```python
from build123d import *

# Parameters (mm, degrees)
F0_W      = 356
F0_H      = 100
F1_DEPTH  = 5
F2_R      = 5
F2_R_2    = 12.5
F3_DEPTH  = 5.001
F4_R      = 1.5
F5_DEPTH  = 5.001
F6_W      = 49.406879
F6_H      = 21.095738
F7_DEPTH  = 25
F9_W      = 63.062
F9_H      = 100
F10_DEPTH = 5
F11_R     = 3
F12_DEPTH = 25
F13_W     = 419.062
F13_H     = 5
F14_DEPTH = 70


with BuildPart() as f1:
    # F0 (on Top) → F1 (new body)
    with BuildSketch(Plane.XY):
        Rectangle(F0_W, F0_H)
    extrude(amount=F1_DEPTH)

    # F2 (on face) → F3 (cut, through all)
    with BuildSketch(Plane.XY.offset(5)):
        with Locations((-155, 37.335402)):
            Circle(F2_R)
        with Locations((155, 37.335402)):
            Circle(F2_R)
        with Locations((-48.086096, 0)):
            Circle(F2_R_2)
        with Locations((51.913904, 0)):
            Circle(F2_R_2)
    extrude(amount=-F3_DEPTH, mode=Mode.SUBTRACT)

    # F4 (on face) → F5 (cut, through all)
    with BuildSketch(Plane.XY.offset(5)):
        with Locations((0, 2.148001)):
            Circle(F4_R)
        with Locations((100, 2.148001)):
            Circle(F4_R)
        with Locations((-100, 2.148001)):
            Circle(F4_R)
    extrude(amount=-F5_DEPTH, mode=Mode.SUBTRACT)

    # F9 (on Top) → F10 (join, through all)
    with BuildSketch(Plane.XY):
        with Locations((-209.531, 0)):
            Rectangle(F9_W, F9_H)
    extrude(amount=F10_DEPTH)

    # F11 (on face) → F12 (cut)
    with BuildSketch(Plane.XY.offset(5)):
        with Locations((-223.56236, -20)):
            Circle(F11_R)
        with Locations((-223.56236, -40)):
            Circle(F11_R)
    extrude(amount=-F12_DEPTH, mode=Mode.SUBTRACT)

    # F13 (on face) → F14 (join)
    with BuildSketch(Plane(origin=(0, 0, 0), x_dir=(1, 0, 0), z_dir=(0, 0, -1))):
        with Locations((-31.531, -52.5)):
            Rectangle(F13_W, F13_H)
    extrude(amount=-F14_DEPTH)


with BuildPart() as f7:
    # F6 (on Top) → F7 (new body)
    with BuildSketch(Plane.XY):
        with Locations((37.024449, 48.380569)):
            Rectangle(F6_W, F6_H)
    extrude(amount=F7_DEPTH)


solid = f1.part
```
The listing builds one solid part. Answer for the finished solid, in the listing's coordinates (mm). A direction names the side the tool comes from. Give positions to 0.01 mm unless a question says otherwise; leave off trailing zeros. Write each loop counter-clockwise with the first axis right and the second up, starting at its lowest first coordinate (ties: lowest second). Pieces come first, ordered by that corner, then holes. Notation, with made-up numbers: (-1, 44) -> (53, 44) arc R28 ccw to (53, 67) -> close; hole circle Ø7 at (74, 59). An arc over 180 degrees is marked (long way). Write item = value, one per line. Start each with the question number.
1) Which of the six approach directions +Z, -Z, +X, -X, +Y, -Y give full straight-line access (tool end or side, diameter ignored) to faces 4 (the face through (-34, 1, 5)), 5 (the face through (-241.062, 18, 4))?
2) The part is cut by section C-C, the plane y = -33. Determine the outline of the cut face in (x, z), and give its area (3 significant figures).
3) The part is cut by section A-A, the plane x = -155. Determine the outline of the cut face in (y, z), and give its area (3 significant figures).
4) The part is cut by section B-B, the plane z = 17.5. Determine the outline of the cut face in (x, y).
5) Straight lines are drawn through the part: line 1 along Y through (x, z) = (155, 2.1); line 2 along Y through (x, z) = (100, 1); line 3 along Y through (x, z) = (152, 24). For each, find the intervals that lie inside material, in ascending order.
6) Determine the mould class of faces 1 (the face through (-34, 50, 37)), 2 (the face through (178, 18, 4)), 3 (the face through (-158.968, 34.293, 2.535)) for opening direction X: +X half, -X half, draft (parallel to the pull), parting line (faces both ways), or undercut.
7) Each of these flat-tipped pins is pushed along its axis until it touches: pin 1 (2.5 mm diameter, centred on x = 0, y = 2.148, fed in from +Z); pin 2 (9.5 mm diameter, centred on x = -223.56, y = -40, fed in from +Z). Where does it stop, or does it pass through?
Solutions:
q1.face_4 = +Z, +X, -X, -Y
q1.face_5 = +Z, -Z, -X, +Y, -Y
q2.outline = (-241.06, 0) -> (178, 0) -> (178, 5) -> (-241.06, 5) -> close
q2.area = 2,100 mm²
q3.outline = (-50, 0) -> (32.34, 0) -> (32.34, 5) -> (-50, 5) -> close; (42.34, 0) -> (55, 0) -> (55, 70) -> (50, 70) -> (50, 5) -> (42.34, 5) -> close
q3.area = 800 mm²
q4.outline = (-241.06, 50) -> (178, 50) -> (178, 55) -> (-241.06, 55) -> close
q5.line_1 = -50 to 32.34, 42.34 to 55
q5.line_2 = -50 to 0.65, 3.65 to 55
q5.line_3 = 50 to 55
q6.face_1 = draft
q6.face_2 = +X half
q6.face_3 = undercut
q7.pin_1 = through
q7.pin_2 = 5
